Autodesk Inventor part; units mm, degrees
ref_plane "YZ Plane" through (0, 0, 0) normal (1, 0, 0) x (0, 1, 0)
ref_plane "XZ Plane" through (0, 0, 0) normal (0, 1, 0) x (-1, 0, 0)
ref_plane "XY Plane" through (0, 0, 0) normal (0, 0, 1) x (1, 0, 0)
sketch "Esquisse1" plane through (0, 0, 0) normal (0, 0, 1) x (1, 0, 0)
  circle A0 centre (0, 0) radius 14.5
  dimension "d0" = 29
extrude "Extrusion1" add sketch "Esquisse1" along normal blind 38.8
sketch "Esquisse2" plane through (0, 0, 38.8) normal (0, 0, 1) x (1, 0, 0)
  circle A0 centre (0, 0) radius 14.5
  circle A1 centre (0, 0) radius 5
  dimension "d3" = 10
extrude "Extrusion2" add sketch "Esquisse2" along normal blind 2.7 contours A1
sketch "Esquisse3" plane through (0, 0, 41.5) normal (0, 0, 1) x (1, 0, 0)
  circle A0 centre (0, 0) radius 5
  circle A1 centre (0, 0) radius 1.25
  dimension "d6" = 2.5
extrude "Extrusion3" add sketch "Esquisse3" along normal blind 9.3 contours A1
sketch "Esquisse4" plane through (0, 0, 0) normal (0, 0, -1) x (-1, 0, 0)
  circle A0 centre (0, 0) radius 14.5
  circle A1 centre (0, 0) radius 5
  dimension "d9" = 10
extrude "Extrusion4" add sketch "Esquisse4" along normal blind 3.2 contours A1
fillet "Congé1" radius 1 1 edges at (-14.5, 0, 38.8)
fillet "Congé2" radius 0.5 1 edges at (-1.25, 0, 50.8)
sketch "Esquisse5" plane through (0, 0, 38.8) normal (0, 0, 1) x (1, 0, 0)
  circle A0 centre (0, 0) radius 5
  circle A1 centre (0, 8) radius 1.3
  circle A2 centre (0, -8) radius 1.3
  dimension "d14" = 2.6
  dimension "d15" = 8
  dimension "d16" = 2.6
  dimension "d17" = 8
extrude "Extrusion5" cut sketch "Esquisse5" against normal blind 3 contours A1 | A2
thread "Filetage1"
thread "Filetage2"
equation "\"d16\" = d14"
equation "\"d17\" = d15"
properties part number "Nidec_DMN29"
Here's how the part is built. I have some questions about the finished solid (model axes, mm). A direction names the side the tool comes from. Give positions to 0.01 mm unless a question says otherwise; leave off trailing zeros. Loops run counter-clockwise (first coordinate to the right, second up) from the corner with the lowest first, then second, coordinate; pieces in that order, holes last. Notation, with made-up numbers: (43, -5.75) -> (101, -5.75) arc R18 ccw to (101, 11.25) -> close; hole circle Ø1 at (-12, -1). An arc over 180 degrees is marked (long way). Answer as a JSON object with one key per item and string values. Group by question number.
Item 1: Imagine slicing it at C-C on z = 47. Write out the boundary of the cut face in (x, y), then the cut area to 3 significant figures.
Item 2: On a 3-axis mill with a long thin cutter (end or side, diameter ignored), from which of +Z, -Z, +X, -X, +Y, -Y can I reach the whole of each face in a straight line? I mean faces 1 (the flat face through (6, 0, 38.8)), 2 (the flat face through (0, 0, 50.8)), 3 (the cylindrical face through (1.08, 4.88, -1.58)). Say none if no direction works.
Item 3: Imagine slicing it at B-B on y = 0. Write out the boundary of the cut face in (x, z).
Item 4: Imagine slicing it at D-D on z = 24. Write out the boundary of the cut face in (x, y).
Item 5: Will these pins go through, and if not, where does the flat tip stop? pin 1 (5 mm diameter, centred on y = -8.5, z = 11, fed in from -X); pin 2 (1.3 mm diameter, centred on x = 0.5, y = -7.5, fed in from +Z); pin 3 (6 mm diameter, centred on y = -8.5, z = 35, fed in from -X).
Item 6: I need wall thicknesses on L1, parallel to Y at x = 0, z = 36.8; L2, parallel to Z at x = -2.25, y = 7; L3, parallel to Y at x = -0.5, z = 5. Which ranges of each line are inside material? Lowest first, please.
Item 7: Thinking about a two-plate mould opening in Y: for faces 4 (the cylindrical face through (6.691, 12.864, 18.635)), 5 (the flat face through (0, 8, 35.8)), 6 (the flat face through (1, -1, 41.5)), which applies, pulls with the +Y half, pulls with the -Y half, needs draft (parallel to the pull), parting line crosses it, or undercut?
Item 8: Imagine slicing it at A-A on x = 0. Write out the boundary of the cut face in (y, z), then the cut area to 3 significant figures.
Answer list:
{
 "1": {"outline": "circle Ø2.5 at (0, 0)", "area": "4.91 mm2"},
 "2": {"face 1": "+Z", "face 2": "+Z, +X, -X, +Y, -Y", "face 3": "-Z"},
 "3": {"outline": "(-14.5, 0) -> (-5, 0) -> (-5, -3.2) -> (5, -3.2) -> (5, 0) -> (14.5, 0) -> (14.5, 37.8) arc R1 ccw to (13.5, 38.8) -> (5, 38.8) -> (5, 41.5) -> (1.25, 41.5) -> (1.25, 50.3) arc R0.5 ccw to (0.75, 50.8) -> (-0.75, 50.8) arc R0.5 ccw to (-1.25, 50.3) -> (-1.25, 41.5) -> (-5, 41.5) -> (-5, 38.8) -> (-13.5, 38.8) arc R1 ccw to (-14.5, 37.8) -> close"},
 "4": {"outline": "circle Ø29 at (0, 0)"},
 "5": {"pin 1": "stops at x = -13.2", "pin 2": "stops at z = 38.8", "pin 3": "stops at x = -13.42"},
 "6": {"L1": "y = -14.5 to -9.3, -6.7 to 6.7, 9.3 to 14.5", "L2": "z = 0 to 38.8", "L3": "y = -14.49 to 14.49"},
 "7": {"face 4": "parting line crosses it", "face 5": "undercut", "face 6": "needs draft"},
 "8": {"outline": "(-14.5, 0) -> (-5, 0) -> (-5, -3.2) -> (5, -3.2) -> (5, 0) -> (14.5, 0) -> (14.5, 37.8) arc R1 ccw to (13.5, 38.8) -> (9.3, 38.8) -> (9.3, 35.8) -> (6.7, 35.8) -> (6.7, 38.8) -> (5, 38.8) -> (5, 41.5) -> (1.25, 41.5) -> (1.25, 50.3) arc R0.5 ccw to (0.75, 50.8) -> (-0.75, 50.8) arc R0.5 ccw to (-1.25, 50.3) -> (-1.25, 41.5) -> (-5, 41.5) -> (-5, 38.8) -> (-6.7, 38.8) -> (-6.7, 35.8) -> (-9.3, 35.8) -> (-9.3, 38.8) -> (-13.5, 38.8) arc R1 ccw to (-14.5, 37.8) -> close", "area": "1,190 mm2"}
}
